Model file for the job. Use its own axes, mm. Coordinates: 2 decimals unless noted, no trailing zeros. Order: outer loops, then holes, each group sorted by start corner. A loop starts at its lowest first (then second) coordinate and runs counter-clockwise, first axis right, second up. Notation, with made-up numbers: M -7.5,78 L 21.5,78 A9 cw 21.5,93 Z; hole C 44,15 d6. An arc over 180 degrees is marked long. Return JSON: item names as keys, results as strings.
```python
from build123d import *

# Parameters (mm, degrees)
SKETCH1_W                                          = 152.4
SKETCH1_H                                          = 25.4
EXTRUDE1_DEPTH                                     = 6.35
F_4_40_TAPPED_HOLE2_D                              = 2.2606
F_4_40_TAPPED_HOLE2_DEPTH                          = 3.302
F_4_40_TAPPED_HOLE2_TIP                            = 0.679152758
F_1_2_0_5_DIAMETER_HOLE1_D                         = 12.7
CSK_FOR_10_FLAT_HEAD_SOCKET_CAP_SCREW2_D           = 5.1054
CSK_FOR_10_FLAT_HEAD_SOCKET_CAP_SCREW2_CSINK_D     = 10.21334
CSK_FOR_10_FLAT_HEAD_SOCKET_CAP_SCREW2_CSINK_ANGLE = 82
CSK_FOR_10_FLAT_HEAD_SOCKET_CAP_SCREW1_D           = 5.1054
CSK_FOR_10_FLAT_HEAD_SOCKET_CAP_SCREW1_CSINK_D     = 10.21334
CSK_FOR_10_FLAT_HEAD_SOCKET_CAP_SCREW1_CSINK_ANGLE = 82


with BuildPart() as part:
    # Sketch1 → Extrude1 (new body)
    with BuildSketch(Plane.XY):
        Rectangle(SKETCH1_W, SKETCH1_H)
    extrude(amount=EXTRUDE1_DEPTH)

    # #4-40 Tapped Hole2
    with Locations(Plane(origin=(-69.85, 0, 6.35), x_dir=(1, 0, 0), z_dir=(0, 0, 1))):
        with Locations((0, 0)):
            Hole(F_4_40_TAPPED_HOLE2_D / 2, depth=F_4_40_TAPPED_HOLE2_DEPTH)
            with Locations((0, 0, -(F_4_40_TAPPED_HOLE2_DEPTH + F_4_40_TAPPED_HOLE2_TIP / 2))):  # 118° drill point
                Cone(0, F_4_40_TAPPED_HOLE2_D / 2, F_4_40_TAPPED_HOLE2_TIP, mode=Mode.SUBTRACT)

    # 1/2 (0.5) Diameter Hole1 (through all)
    with Locations(Plane(origin=(25.4, 0, 6.35), x_dir=(1, 0, 0), z_dir=(0, 0, 1))):
        with Locations((0, 0)):
            Hole(F_1_2_0_5_DIAMETER_HOLE1_D / 2)

    # CSK for #10 Flat Head Socket Cap Screw2 (through all)
    with Locations(Plane(origin=(-2.296155795, -5.361260674, 6.35), x_dir=(1, 0, 0), z_dir=(0, 0, 1))):
        with Locations((59.446155795, 5.361260674)):
            CounterSinkHole(CSK_FOR_10_FLAT_HEAD_SOCKET_CAP_SCREW2_D / 2, CSK_FOR_10_FLAT_HEAD_SOCKET_CAP_SCREW2_CSINK_D / 2, counter_sink_angle=CSK_FOR_10_FLAT_HEAD_SOCKET_CAP_SCREW2_CSINK_ANGLE)

    # CSK for #10 Flat Head Socket Cap Screw1 (through all)
    with Locations(Plane(origin=(-2.296155795, -5.361260674, 6.35), x_dir=(1, 0, 0), z_dir=(0, 0, 1))):
        with Locations((-48.503844205, 5.361260674)):
            CounterSinkHole(CSK_FOR_10_FLAT_HEAD_SOCKET_CAP_SCREW1_D / 2, CSK_FOR_10_FLAT_HEAD_SOCKET_CAP_SCREW1_CSINK_D / 2, counter_sink_angle=CSK_FOR_10_FLAT_HEAD_SOCKET_CAP_SCREW1_CSINK_ANGLE)


solid = part.part
```
Item 1: Saw through at A-A (x = 25.4). Write the cut outline in (y, z).
Check result:
{"outline": "M -12.7,0 L -6.35,0 L -6.35,6.35 L -12.7,6.35 Z; M 6.35,0 L 12.7,0 L 12.7,6.35 L 6.35,6.35 Z"}
Item 2: Pull direction X, two halves, no side cores. Call faces 1 (the flat face through (-76.2, 0, 3)), 2 (the conical face through (59.82, 0.12, 3.55)), 3 (the cylindrical face through (54.715, 0.767, 1.682)), 4 (the flat face through (-1, 0, 6.35)): +X half, -X half, draft (parallel to the pull), parting line (faces both ways), or undercut.
Check result:
{"face 1": "-X half", "face 2": "undercut", "face 3": "undercut", "face 4": "draft"}
Item 3: Wall check: line 1 (Y direction, x = 25.4, z = 2.5); line 2 (X direction, y = -1.75, z = 5); line 3 (Y direction, x = 57.15, z = 1.5). Give the ranges that are in metal, low to high.
Check result:
{"line 1": "y = -12.7 to -6.35, 6.35 to 12.7", "line 2": "x = -76.2 to -54.32, -47.28 to 19.3, 31.5 to 53.63, 60.67 to 76.2", "line 3": "y = -12.7 to -2.55, 2.55 to 12.7"}
Item 4: Saw through at B-B (x = -50.8). Write the cut outline in (y, z).
Check result:
{"outline": "M -12.7,0 L -2.55,0 L -2.55,3.41 L -5.11,6.35 L -12.7,6.35 Z; M 2.55,0 L 12.7,0 L 12.7,6.35 L 5.11,6.35 L 2.55,3.41 Z"}
